Verification items for this drawing (mm, ordinates from the low corner). A direction names the side the tool comes from. Round coordinates to 2 decimals unless told otherwise and drop trailing zeros. Loops run counter-clockwise (first coordinate to the right, second up) from the corner with the lowest first, then second, coordinate; pieces in that order, holes last. Notation, with made-up numbers: (-22.5, -4) - (-4.5, -4) arc R38 ccw to (-4.5, 35) - close; hole circle Ø8 at (-19.75, 15.25). An arc over 180 degrees is marked (long way). Put each result on its own line as item: value. Start each with the question number.
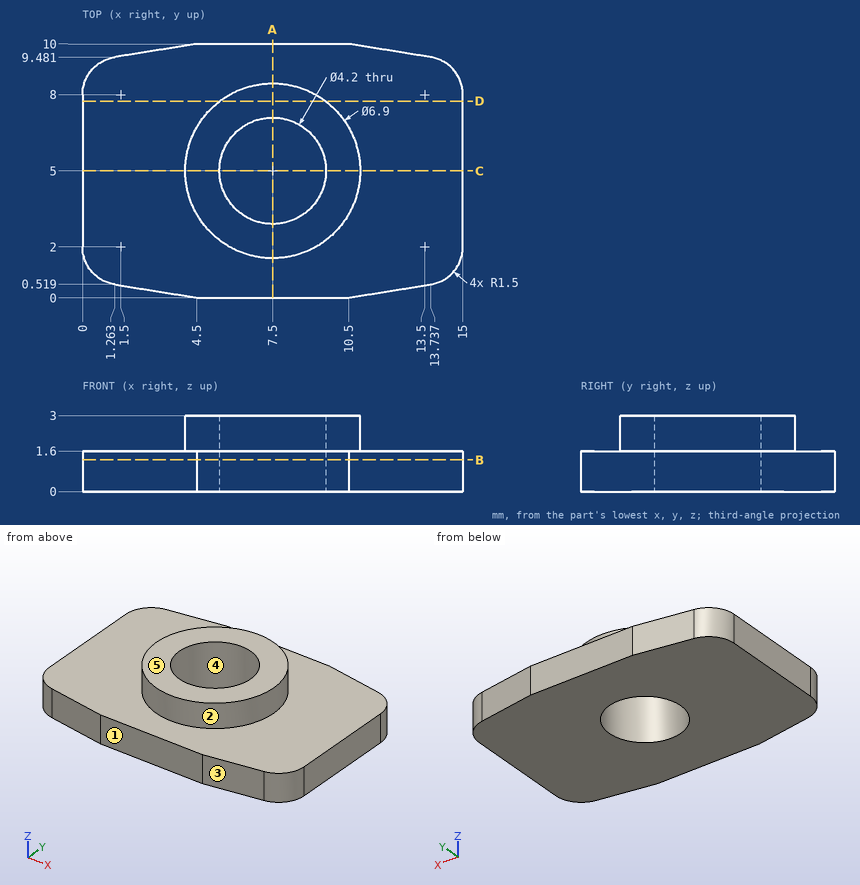
Q1. Material ranges on line 1 (Y direction, x = 7.5, z = 2.3); line 2 (Y direction, x = 13.75, z = 0.2); line 3 (Z direction, x = 3.75, y = 8.25), recorded low to high. Write a range as from..to.
Q2. Draft check along X on the marked faces 3, 4 and 5. Enter one of: +X half, -X half, draft (parallel to the pull), parting line (faces both ways), or undercut.
Q3. Set-up check for the marked faces 1 and 2: record each of +Z, -Z, +X, -X, +Y, -Y from which the full face is reachable in a straight line by a thin tool's end or side.
Q4. Cross-section at B-B on z = 1.25. Enter the section's corners in (x, y).
Q5. Cross-section at A-A on x = 7.5. Enter the section's corners in (y, z).
Q6. Cross-section at D-D on y = 7.75. Enter the section's corners in (x, z).
Q7. Depth check by flat-ended pin: pin 1 Ø6 at (x, y) = (12.5, 2.5) entering from +Z. Enter the tip coordinate at first touch or a pass-through.
Q8. Cross-section at C-C on y = 5. Enter the section's corners in (x, z).
Answer list:
1. line 1: y = 1.55..2.9, 7.1..8.45
1. line 2: y = 0.52..9.48
1. line 3: z = 0..1.6
2. face 3: +X half
2. face 4: undercut
2. face 5: draft
3. face 1: +Z, -Z, +X, -X, -Y
3. face 2: +Z
4. outline: (0, 2) arc R1.5 ccw to (1.26, 0.52) - (4.5, 0) - (10.5, 0) - (13.74, 0.52) arc R1.5 ccw to (15, 2) - (15, 8) arc R1.5 ccw to (13.74, 9.48) - (10.5, 10) - (4.5, 10) - (1.26, 9.48) arc R1.5 ccw to (0, 8) - close; hole circle Ø4.2 at (7.5, 5)
5. outline: (0, 0) - (2.9, 0) - (2.9, 3) - (1.55, 3) - (1.55, 1.6) - (0, 1.6) - close; (7.1, 0) - (10, 0) - (10, 1.6) - (8.45, 1.6) - (8.45, 3) - (7.1, 3) - close
6. outline: (0, 0) - (15, 0) - (15, 1.6) - (9.58, 1.6) - (9.58, 3) - (5.42, 3) - (5.42, 1.6) - (0, 1.6) - close
7. pin 1: stops at z = 3
8. outline: (0, 0) - (5.4, 0) - (5.4, 3) - (4.05, 3) - (4.05, 1.6) - (0, 1.6) - close; (9.6, 0) - (15, 0) - (15, 1.6) - (10.95, 1.6) - (10.95, 3) - (9.6, 3) - close
